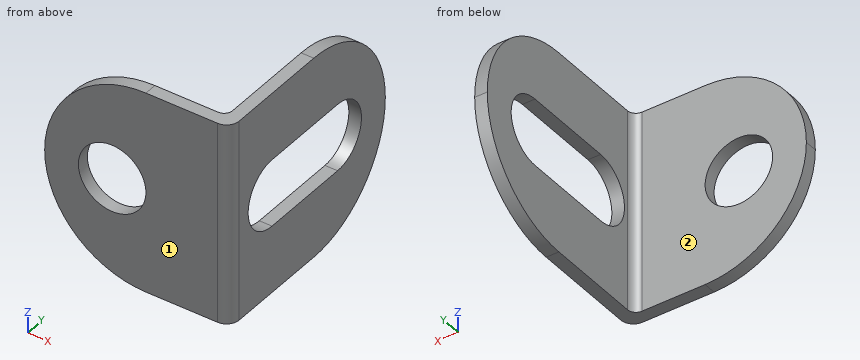
from build123d import *

# Parameters (mm, degrees)
ESTRUSIONE_SOTTILE1_DEPTH = 6
RACCORDO3_R               = 6
SCHIZZO4_R                = 2
TAGLIO_ESTRUSIONE1_DEPTH  = 0.75
RACCORDO1_R               = 0.75
RACCORDO2_R               = 0.5
TAGLIO_ESTRUSIONE2_DEPTH  = 0.75


with BuildPart() as part:
    # Schizzo1 → Estrusione-Sottile1 (new, symmetric)
    with BuildSketch(Plane.XY):
        Polygon((0, 13), (0, 0), (-11, 0), (-11, 0.75), (-0.75, 0.75), (-0.75, 13), align=None)
    extrude(amount=ESTRUSIONE_SOTTILE1_DEPTH, both=True)

    # Raccordo3
    raccordo3_edges = [part.edges().sort_by_distance(p)[0] for p in [
        (-11, 0.375, 6),
        (-11, 0.375, -6),
        (-0.375, 13, -6),
        (-0.375, 13, 6),
    ]]
    fillet(raccordo3_edges, radius=RACCORDO3_R - 0.0001)  # a hair under: the kernel refuses the full size

    # Schizzo4 → Taglio-Estrusione1 (cut)
    with BuildSketch(Plane(origin=(0, 0.75, 0), x_dir=(1, 0, 0), z_dir=(0, 1, 0))):
        with Locations(Location((-7, 0, 0), (0, 0, 180))):
            Circle(SCHIZZO4_R)
    extrude(amount=-TAGLIO_ESTRUSIONE1_DEPTH, mode=Mode.SUBTRACT)

    # Raccordo1
    raccordo1_edges = [part.edges().sort_by_distance(p)[0] for p in [
        (0, 0, 0),
    ]]
    fillet(raccordo1_edges, radius=RACCORDO1_R)

    # Raccordo2
    raccordo2_edges = [part.edges().sort_by_distance(p)[0] for p in [
        (-0.75, 0.75, 0),
    ]]
    fillet(raccordo2_edges, radius=RACCORDO2_R)

    # Schizzo5 → Taglio-Estrusione2 (cut)
    with BuildSketch(Plane.ZY.offset(0.75)):
        with BuildLine():
            Line((2, 9), (2, 3.5))
            ThreePointArc((2, 3.5), (0, 1.5), (-2, 3.5))
            Line((-2, 3.5), (-2, 9))
            ThreePointArc((-2, 9), (0, 11), (2, 9))
        make_face()
    extrude(amount=-TAGLIO_ESTRUSIONE2_DEPTH, mode=Mode.SUBTRACT)


solid = part.part
Input: part model. Units: mm. Frame: model coordinates. Face numbers are marked on the shaded views. A direction names the side the tool comes from. Give positions to 0.01 mm unless a question says otherwise; leave off trailing zeros. Loops run counter-clockwise (first coordinate to the right, second up) from the corner with the lowest first, then second, coordinate; pieces in that order, holes last. Notation, with made-up numbers: M 58.25,88.25 L 82.25,88.25 A23 ccw 82.25,96.25 Z; hole C 15.5,88 d2. An arc over 180 degrees is marked long. Use one line per item in the form item = value.
1. First-contact query: pin 1 (5 mm diameter, centred on y = 4, z = -2.5, fed in from -X); pin 2 (3 mm diameter, centred on x = -4.5, z = 0, fed in from +Y); pin 3 (5 mm diameter, centred on y = 2.5, z = -3.5, fed in from -X). Flat tips, straight axial feed; report the tip coordinate or a pass-through.
Numbers:
pin_1 = -0.75
pin_2 = 0.75
pin_3 = -10.75
2. Reachability of the marked faces 1 and 2 from +Z, -Z, +X, -X, +Y, -Y: full face, straight path, thin tool, end or side. Return the list, or none.
Numbers:
face_1 = +Z, -Z, +X, -X, -Y
face_2 = +Z, -Z, -X, +Y
3. Section query B-B, the plane x = -7. Return the cut outline in (y, z), and give its area (3 significant figures).
Numbers:
outline = M 0,-5.66 L 0.75,-5.66 L 0.75,-2 L 0,-2 Z; M 0,2 L 0.75,2 L 0.75,5.66 L 0,5.66 Z
area = 5.49 mm²
4. Section query C-C, the plane z = -0.75. Return the cut outline in (x, y), and give its area (3 significant figures).
Numbers:
outline = M -10.95,0 L -8.85,0 L -8.85,0.75 L -10.95,0.75 Z; M -5.15,0 L -0.75,0 A0.75 ccw 0,0.75 L 0,1.65 L -0.75,1.65 L -0.75,1.25 A0.5 cw -1.25,0.75 L -5.15,0.75 Z; M -0.75,10.85 L 0,10.85 L 0,12.95 L -0.75,12.95 Z
area = 7.61 mm²
5. Section query A-A, the plane y = 6. Return the cut outline in (x, z).
Numbers:
outline = M -0.75,-6 L 0,-6 L 0,-2 L -0.75,-2 Z; M -0.75,2 L 0,2 L 0,6 L -0.75,6 Z
6. Section query D-D, the plane z = -2.5. Return the cut outline in (x, y).
Numbers:
outline = M -10.45,0 L -0.75,0 A0.75 ccw 0,0.75 L 0,12.45 L -0.75,12.45 L -0.75,1.25 A0.5 cw -1.25,0.75 L -10.45,0.75 Z
7. Line query: L1, parallel to Y at x = -4, z = -0.75; L2, parallel to Z at x = -7, y = 0.5; L3, parallel to Z at x = -0.5, y = 5.5. Output: solid intervals per line, ascending.
Numbers:
L1 = 0 to 0.75
L2 = -5.66 to -2, 2 to 5.66
L3 = -6 to -2, 2 to 6
